Job drawing, mm, ordinate dimensions from the low corner. One solid piece. A direction names the side the tool comes from. Round coordinates to 2 decimals unless told otherwise and drop trailing zeros. Write each loop counter-clockwise with the first axis right and the second up, starting at its lowest first coordinate (ties: lowest second). Pieces come first, ordered by that corner, then holes. Notation, with made-up numbers: M 16,25.25 L 27,25.25 A17 ccw 27,42.25 Z; hole C -40,23.25 d9. An arc over 180 degrees is marked long. Write each question's results on one line, items separated by ' | '. Start each with the question number.
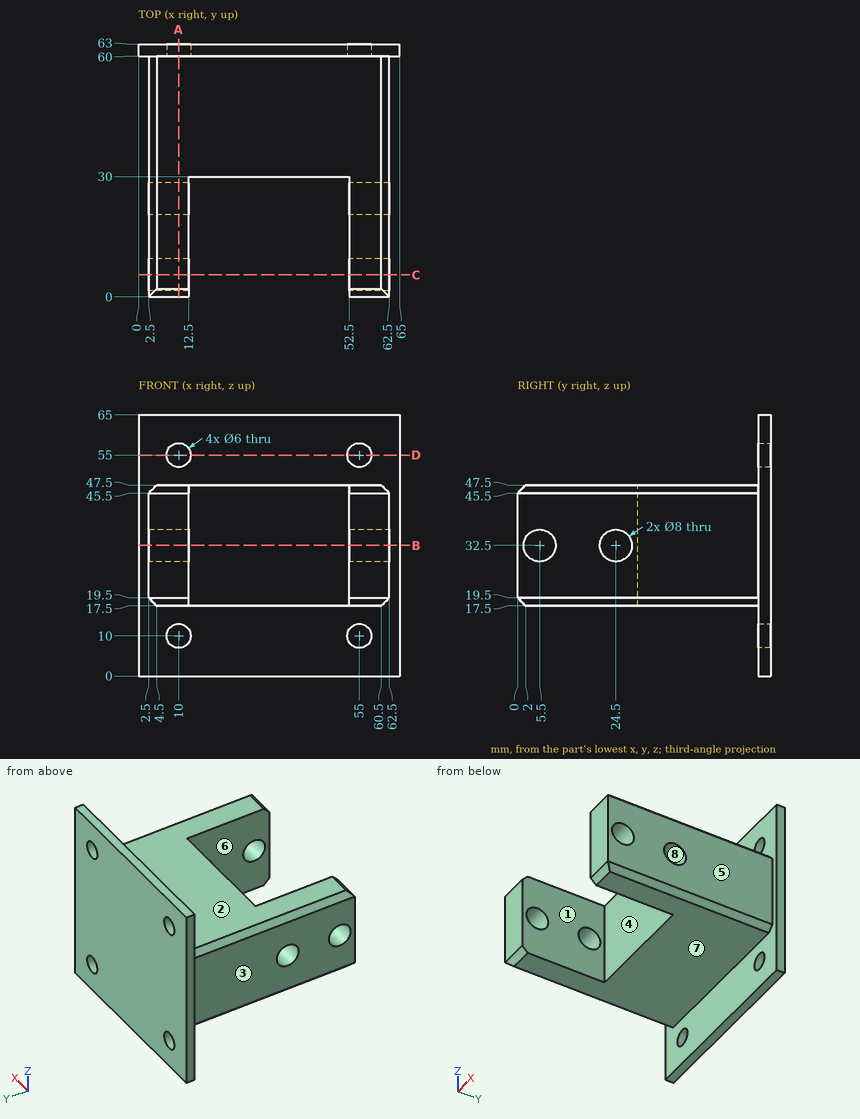
1) Drop flat-ended pins along their axis: pin 1 Ø7 at (x, z) = (55, 10) entering from -Y; pin 2 Ø4 at (x, y) = (10, 14) entering from -Z; pin 3 Ø9 at (y, z) = (13, 40) entering from +X. Give the stop position or say it passes through.
2) 3-axis set-ups, long thin cutter, end or side, ignore diameter. For the marked faces 5, 6, 7 and 8: which of +Z, -Z, +X, -X, +Y, -Y reach the whole face in a straight line?
3) Pull direction X, two halves, no side cores. Call the marked faces 1, 2, 3 and 4: pulls with the +X half, pulls with the -X half, needs draft (parallel to the pull), parting line crosses it, or undercut.
4) Saw through at D-D, the plane z = 55. Write the cut outline in (x, y), plus the area to 3 significant figures.
5) Saw through at A-A, the plane x = 10. Write the cut outline in (y, z), plus the area to 3 significant figures.
6) Wall check: line 1 along Y through (x, z) = (8.75, 32.5); line 2 along X through (y, z) = (61, 55); line 3 along X through (y, z) = (15, 40). Give the ranges that are in metal, low to high. Write a range as from..to.
7) Saw through at C-C, the plane y = 5.5. Write the cut outline in (x, z), plus the area to 3 significant figures.
8) Saw through at B-B, the plane z = 32.5. Write the cut outline in (x, y), plus the area to 4 significant figures.
Filled sheet:
1) pin 1: stops at y = 60 | pin 2: stops at z = 17.5 | pin 3: stops at x = 62.5
2) face 5: +Z, -Z, +X, -Y | face 6: +Z, -Z, -Y | face 7: -Z, +X, -X, -Y | face 8: +X, -X
3) face 1: undercut | face 2: needs draft | face 3: pulls with the -X half | face 4: undercut
4) outline: M 0,60 L 7,60 L 7,63 L 0,63 Z; M 13,60 L 52,60 L 52,63 L 13,63 Z; M 58,60 L 65,60 L 65,63 L 58,63 Z | area: 159 mm^2
5) outline: M 0,19.5 L 2,17.5 L 60,17.5 L 60,13 L 63,13 L 63,52 L 60,52 L 60,47.5 L 2,47.5 L 0,45.5 Z; M 60,0 L 63,0 L 63,7 L 60,7 Z; M 60,58 L 63,58 L 63,65 L 60,65 Z; hole C 5.5,32.5 d8; hole C 24.5,32.5 d8 | area: 1,850 mm^2
6) line 1: y = 0..1.5, 9.5..20.5, 28.5..63 | line 2: x = 0..7, 13..52, 58..65 | line 3: x = 2.5..12.5, 52.5..62.5
7) outline: M 2.5,19.5 L 4.5,17.5 L 12.5,17.5 L 12.5,28.5 L 2.5,28.5 Z; M 2.5,36.5 L 12.5,36.5 L 12.5,47.5 L 4.5,47.5 L 2.5,45.5 Z; M 52.5,17.5 L 60.5,17.5 L 62.5,19.5 L 62.5,28.5 L 52.5,28.5 Z; M 52.5,36.5 L 62.5,36.5 L 62.5,45.5 L 60.5,47.5 L 52.5,47.5 Z | area: 432 mm^2
8) outline: M 0,60 L 2.5,60 L 2.5,28.5 L 12.5,28.5 L 12.5,30 L 52.5,30 L 52.5,28.5 L 62.5,28.5 L 62.5,60 L 65,60 L 65,63 L 0,63 Z; M 2.5,0 L 12.5,0 L 12.5,1.5 L 2.5,1.5 Z; M 2.5,9.5 L 12.5,9.5 L 12.5,20.5 L 2.5,20.5 Z; M 52.5,0 L 62.5,0 L 62.5,1.5 L 52.5,1.5 Z; M 52.5,9.5 L 62.5,9.5 L 62.5,20.5 L 52.5,20.5 Z | area: 2,275 mm^2
